Work out the finished part from the listing and answer in its coordinate system (mm). A direction names the side the tool comes from. Coordinates: 2 decimals unless noted, no trailing zeros. Write each loop counter-clockwise with the first axis right and the second up, starting at its lowest first coordinate (ties: lowest second). Pieces come first, ordered by that corner, then holes. Notation, with made-up numbers: (4.25, -8) - (24.25, -8) arc R17 cw to (24.25, 2) - close; hole circle Ø9 at (85.5, 59). An arc over 180 degrees is marked (long way). Answer as a JSON object with one key per item and string values. Group by question number.
from build123d import *

# Parameters (mm, degrees)
F2_SIZE2 = 0.5
F2_SIZE  = 0.5


with BuildPart() as f1:
    # F0 (on Top) → F1 (revolve)
    with BuildSketch(Plane.XY):
        Polygon((0, 20), (0, 15), (6, 15), (6, 10), (9, 10), (9, 15), (17, 15), (17, 18), (11, 18), (11, 20), align=None)
    revolve(axis=Axis((8.5, 0, 0), (1, 0, 0)))

    # F2
    f2_edges = [f1.edges().sort_by_distance(p)[0] for p in [
        (0, -20, 0),
        (11, -20, 0),
        (17, -18, 0),
        (0, -15, 0),
        (6, -10, 0),
        (9, -10, 0),
        (17, -15, 0),
    ]]
    chamfer(f2_edges, length=F2_SIZE, length2=F2_SIZE2)


solid = f1.part
Q1. Section C-C on x = 8 is taken. Determine the outline of the cut face in (y, z).
Q2. Flat-ended cylindrical pins translate along their axes: pin 1 Ø1.5 at (y, z) = (9, -6.5) entering from +X; pin 2 Ø10 at (x, z) = (13.5, 11.5) entering from +Y; pin 3 Ø8 at (y, z) = (13.5, 0.5) entering from -X; pin 4 Ø2 at (y, z) = (0, -13.5) entering from -X. Find the tip coordinate at first contact, or state that the pin passes through.
Q3. Consider L1, parallel to Z at x = 7, y = 0; L2, parallel to Z at x = 3.3, y = 0; L3, parallel to X at y = -10, z = -15. Determine where each line is inside the solid, lowest interval first. Write a range as from..to.
Q4. A tool of negligible diameter and unlimited length cuts with its end or side. For faces 4 (the face through (5.43, -4.336, -19.524)), 5 (the face through (9, -3.1, 10.2)), 6 (the face through (6, 3.1, 10.2)), from which of +Z, -Z, +X, -X, +Y, -Y can it reach the whole face along a straight path? Write none if from no direction.
Q5. Section D-D on x = 15.75 is taken. Determine the outline of the cut face in (y, z), plus the area to 3 significant figures.
Q6. For a pull along Z with two mould halves and no side action, classify faces 1 (the face through (11, -5.69, -17.24)), 2 (the face through (13.712, -2.343, 17.847)), 3 (the face through (3.288, -14.985, 0.66)) as +Z half, -Z half, draft (parallel to the pull), parting line (faces both ways), or undercut.
Numbers:
{
 "1": {"outline": "circle Ø40 at (0, 0); hole circle Ø20 at (0, 0)"},
 "2": {"pin 1": "stops at x = 9", "pin 2": "stops at y = 18.54", "pin 3": "stops at x = 0", "pin 4": "stops at x = 6"},
 "3": {"L1": "z = -20..-10, 10..20", "L2": "z = -20..-15, 15..20", "L3": "x = 0..11"},
 "4": {"face 4": "+X, -X", "face 5": "+X", "face 6": "-X"},
 "5": {"outline": "circle Ø36 at (0, 0); hole circle Ø30 at (0, 0)", "area": "311 mm²"},
 "6": {"face 1": "draft", "face 2": "parting line", "face 3": "undercut"}
}
